```python
from build123d import *

# Parameters (mm, degrees)
SKETCH1_W               = 100
SKETCH1_H               = 60
BOSS_EXTRUDE1_DEPTH     = 5
SKETCH3_W               = 43.5
SKETCH3_H               = 43.5
CUT_EXTRUDE1_DEPTH      = 1
SKETCH4_R               = 1.75
CUT_EXTRUDE3_DEPTH      = 92
CUT_EXTRUDE3_DEPTH_BACK = 1
SKETCH5_R               = 5
CUT_EXTRUDE4_DEPTH      = 3
SKETCH6_R               = 4
CUT_EXTRUDE5_DEPTH      = 1
CUT_EXTRUDE5_DEPTH_BACK = 6
SKETCH7_R               = 7.5
CUT_EXTRUDE6_DEPTH      = 3
CHAMFER1_SIZE           = 0.5
CHAMFER2_SIZE           = 5
CHAMFER3_SIZE           = 0.5


with BuildPart() as part:
    # Sketch1 → Boss-Extrude1 (new body)
    with BuildSketch(Plane.XY):
        Rectangle(SKETCH1_W, SKETCH1_H)
    extrude(amount=BOSS_EXTRUDE1_DEPTH)

    # Sketch3 → Cut-Extrude1 (cut)
    with BuildSketch(Plane.XY):
        Rectangle(SKETCH3_W, SKETCH3_H)
    extrude(amount=CUT_EXTRUDE1_DEPTH, mode=Mode.SUBTRACT)

    # Sketch4 → Cut-Extrude3 (cut, two sides)
    with BuildSketch(Plane.XY.offset(-48)) as cut_extrude3_sk:
        with Locations((-15.5, 15.5)):
            Circle(SKETCH4_R)
        with Locations((15.5, 15.5)):
            Circle(SKETCH4_R)
        with Locations((15.499999999, -15.5)):
            Circle(SKETCH4_R)
        with Locations((-15.5, -15.5)):
            Circle(SKETCH4_R)
    extrude(amount=CUT_EXTRUDE3_DEPTH, mode=Mode.SUBTRACT)
    extrude(cut_extrude3_sk.sketch, amount=-CUT_EXTRUDE3_DEPTH_BACK, mode=Mode.SUBTRACT)

    # Sketch5 → Cut-Extrude4 (cut)
    with BuildSketch(Plane.XY.offset(5)):
        with Locations((-15.5, 15.5)):
            Circle(SKETCH5_R)
        with Locations((15.5, 15.5)):
            Circle(SKETCH5_R)
        with Locations((15.499999999, -15.5)):
            Circle(SKETCH5_R)
        with Locations((-15.5, -15.5)):
            Circle(SKETCH5_R)
    extrude(amount=-CUT_EXTRUDE4_DEPTH, mode=Mode.SUBTRACT)

    # Sketch6 → Cut-Extrude5 (cut, two sides)
    with BuildSketch(Plane(origin=(0, 0, 0), x_dir=(-1, 0, 0), z_dir=(0, 0, -1))) as cut_extrude5_sk:
        with Locations((-38, 0)):
            Circle(SKETCH6_R)
        with Locations((38, 0)):
            Circle(SKETCH6_R)
    extrude(amount=CUT_EXTRUDE5_DEPTH, mode=Mode.SUBTRACT)
    extrude(cut_extrude5_sk.sketch, amount=-CUT_EXTRUDE5_DEPTH_BACK, mode=Mode.SUBTRACT)

    # Sketch7 → Cut-Extrude6 (cut)
    with BuildSketch(Plane(origin=(0, 0, 0), x_dir=(-1, 0, 0), z_dir=(0, 0, -1))):
        with Locations((-38, 0)):
            Circle(SKETCH7_R)
        with Locations((38, 0)):
            Circle(SKETCH7_R)
    extrude(amount=-CUT_EXTRUDE6_DEPTH, mode=Mode.SUBTRACT)

    # Chamfer1
    chamfer1_edges = [part.edges().sort_by_distance(p)[0] for p in [
        (45.5, 0, 0),
        (-30.5, 0, 0),
    ]]
    chamfer(chamfer1_edges, length=CHAMFER1_SIZE)

    # Chamfer2
    chamfer2_edges = [part.edges().sort_by_distance(p)[0] for p in [
        (50, -30, 2.5),
        (-50, -30, 2.5),
        (-50, 30, 2.5),
        (50, 30, 2.5),
    ]]
    chamfer(chamfer2_edges, length=CHAMFER2_SIZE)

    # Chamfer3
    chamfer3_edges = [part.edges().sort_by_distance(p)[0] for p in [
        (0, 30, 0),
        (50, 0, 0),
        (0, -30, 0),
        (-50, 0, 0),
        (47.5, -27.5, 0),
        (-47.5, -27.5, 0),
        (-47.5, 27.5, 0),
        (47.5, 27.5, 0),
    ]]
    chamfer(chamfer3_edges, length=CHAMFER3_SIZE)


solid = part.part
```
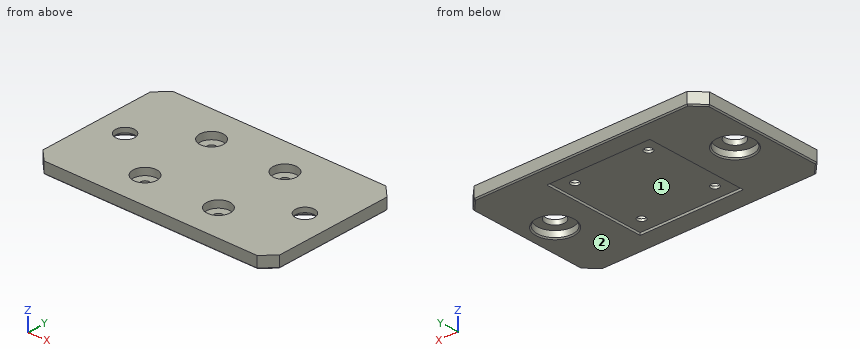
For this review, take the finished solid that the model builds, in its own axes (mm). Face numbers are marked on the shaded views. Coordinates: 2 decimals unless noted, no trailing zeros. Write each loop counter-clockwise with the first axis right and the second up, starting at its lowest first coordinate (ties: lowest second). Pieces come first, ordered by that corner, then holes. Notation, with made-up numbers: (-7.75, -29) - (-2.75, -29) arc R29 cw to (-2.75, 2) - close; hole circle Ø8 at (77, 17). An arc over 180 degrees is marked (long way). Put each result on its own line as item: value.
1. Add section A-A, the plane y = -15.5. Give the boundary of the cut face in (x, z).
Values found:
outline: (-50, 0.5) - (-49.5, 0) - (-21.75, 0) - (-21.75, 1) - (-17.25, 1) - (-17.25, 2) - (-20.5, 2) - (-20.5, 5) - (-50, 5) - close; (-13.75, 1) - (13.75, 1) - (13.75, 2) - (10.5, 2) - (10.5, 5) - (-10.5, 5) - (-10.5, 2) - (-13.75, 2) - close; (17.25, 1) - (21.75, 1) - (21.75, 0) - (49.5, 0) - (50, 0.5) - (50, 5) - (20.5, 5) - (20.5, 2) - (17.25, 2) - close
2. Wall thickness on probe 1 along Y at (x, z) = (15.5, 1.45); probe 2 along Y at (x, z) = (-38, 1.4); probe 3 along Y at (x, z) = (16, 0.75): over which ranges is each line inside the solid? List them lowest first.
Values found:
probe 1: -30 to -17.25, -13.75 to 13.75, 17.25 to 30
probe 2: -30 to -7.5, 7.5 to 30
probe 3: -30 to -21.75, 21.75 to 30
3. Add section C-C, the plane x = 38. Give the boundary of the cut face in (y, z).
Values found:
outline: (-30, 0.5) - (-29.5, 0) - (-8, 0) - (-7.5, 0.5) - (-7.5, 3) - (-4, 3) - (-4, 5) - (-30, 5) - close; (4, 3) - (7.5, 3) - (7.5, 0.5) - (8, 0) - (29.5, 0) - (30, 0.5) - (30, 5) - (4, 5) - close
4. Mouldability with a two-part tool opening along Y and no side actions: class the marked faces 1 and 2 as released by +Y, released by -Y, zero draft, split by the parting line, or undercut.
Values found:
face 1: undercut
face 2: zero draft
5. For pin 1 (12 mm diameter, centred on x = -36, y = -0.5, fed in from -Z); pin 2 (4.5 mm diameter, centred on x = -15.5, y = -15.5, fed in from +Z); pin 3 (4 mm diameter, centred on x = 15.5, y = -15.5, fed in from -Z), all flat-tipped, find the tip position at first contact; note any pin that passes through.
Values found:
pin 1: z = 0
pin 2: z = 2
pin 3: z = 1
6. Add section B-B, the plane x = 15.5. Give the boundary of the cut face in (y, z).
Values found:
outline: (-30, 0.5) - (-29.5, 0) - (-21.75, 0) - (-21.75, 1) - (-17.25, 1) - (-17.25, 2) - (-20.5, 2) - (-20.5, 5) - (-30, 5) - close; (-13.75, 1) - (13.75, 1) - (13.75, 2) - (10.5, 2) - (10.5, 5) - (-10.5, 5) - (-10.5, 2) - (-13.75, 2) - close; (17.25, 1) - (21.75, 1) - (21.75, 0) - (29.5, 0) - (30, 0.5) - (30, 5) - (20.5, 5) - (20.5, 2) - (17.25, 2) - close
7. Add section D-D, the plane y = -9. Give the boundary of the cut face in (x, z).
Values found:
outline: (-50, 0.5) - (-49.5, 0) - (-21.75, 0) - (-21.75, 1) - (21.75, 1) - (21.75, 0) - (49.5, 0) - (50, 0.5) - (50, 5) - (-50, 5) - close
